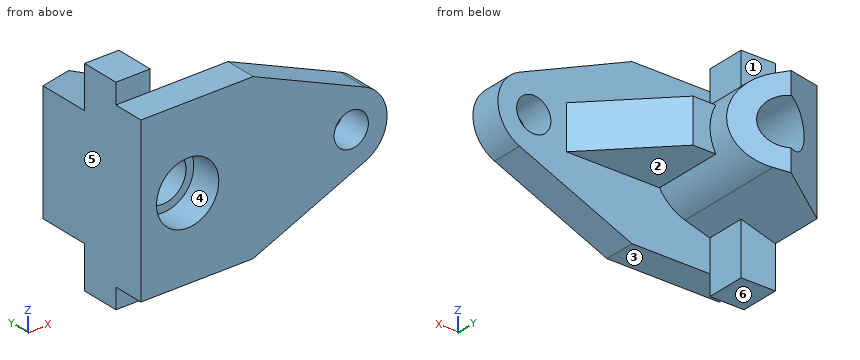
from build123d import *

# Parameters (mm, degrees)
BOSS_EXTRUDE2_DEPTH = 10
SKETCH2_R           = 5.5
CUT_EXTRUDE1_DEPTH  = 10
SKETCH3_W           = 11
SKETCH3_H           = 65
BOSS_EXTRUDE3_DEPTH = 12.5
BOSS_EXTRUDE4_START = -10
BOSS_EXTRUDE4_DEPTH = 47.5
SKETCH7_R           = 7.5
CUT_EXTRUDE2_DEPTH  = 89.705974996
RIB1_START          = -7
RIB1_DEPTH          = 14
CUT_EXTRUDE3_START  = -19
CUT_EXTRUDE3_DEPTH  = 38


# Read off the part's stored shape, not the designer's step: Rib1, Cut-Extrude3
with BuildPart() as part:
    # Sketch1 → Boss-Extrude2 (new body)
    with BuildSketch(Plane(origin=(0, 0, 0), x_dir=(1, 0, 0), z_dir=(0, 1, 0))):
        with BuildLine():
            Line((-67.5, 26), (-67.5, -26))
            Line((-67.5, -26), (-31.5, -26))
            Line((-31.5, -26), (4.527189528, -10.571402697))
            ThreePointArc((4.527189528, -10.571402697), (11.5, 0), (4.527189528, 10.571402697))
            Line((4.527189528, 10.571402697), (-31.5, 26))
            Line((-31.5, 26), (-67.5, 26))
        make_face()
    extrude(amount=BOSS_EXTRUDE2_DEPTH)

    # Sketch2 → Cut-Extrude1 (cut)
    with BuildSketch(Plane(origin=(0, 10, 0), x_dir=(1, 0, 0), z_dir=(0, 1, 0))):
        with Locations(Location((0, 0, 0), (0, 0, 270))):
            Circle(SKETCH2_R)
    extrude(amount=-CUT_EXTRUDE1_DEPTH, mode=Mode.SUBTRACT)

    # Sketch3 → Boss-Extrude3 (add)
    with BuildSketch(Plane(origin=(0, 10, 0), x_dir=(1, 0, 0), z_dir=(0, 1, 0))):
        with Locations((-62, 0)):
            Rectangle(SKETCH3_W, SKETCH3_H)
    extrude(amount=BOSS_EXTRUDE3_DEPTH)

    # Sketch4 → Boss-Extrude4 (add)
    with BuildSketch(Plane(origin=(0, 10, 0), x_dir=(1, 0, 0), z_dir=(0, 1, 0)).offset(BOSS_EXTRUDE4_START)):
        with BuildLine():
            Line((-67.5, 19), (-67.5, -19))
            Line((-67.5, -19), (-48.552766046, -13.432026806))
            ThreePointArc((-48.552766046, -13.432026806), (-38.5, 0), (-48.552766046, 13.432026806))
            Line((-48.552766046, 13.432026806), (-67.5, 19))
        make_face()
    extrude(amount=BOSS_EXTRUDE4_DEPTH)

    # Sketch6 → Hole1 (revolve, cut)
    with BuildSketch(Plane(origin=(-52.5, 10, 0), x_dir=(0, 0, 1), z_dir=(1, 0, 0))):
        Polygon((0, 0), (0, 10), (7, 10), (7, 15), (10, 15), (10, 0), align=None)
    revolve(axis=Axis((-52.5, -100, 0), (0, 1, 0)), mode=Mode.SUBTRACT)

    # Sketch7 → Cut-Extrude2 (cut, through all)
    with BuildSketch(Plane(origin=(0, 47.5, 0), x_dir=(1, 0, 0), z_dir=(0, 1, 0))):
        with Locations(Location((-52.5, 0, 0), (0, 0, 270))):
            Circle(SKETCH7_R)
    extrude(amount=-CUT_EXTRUDE2_DEPTH, mode=Mode.SUBTRACT)

    # Rib1 outline → Rib1 (add)
    with BuildSketch(Plane.XY.offset(RIB1_START)):
        Polygon((-33, 32.5), (-42, 32.5), (-42, 10), (-10.5, 10), align=None)
    extrude(amount=RIB1_DEPTH)

    # Cut-Extrude3 outline → Cut-Extrude3 (cut)
    with BuildSketch(Plane.XY.offset(CUT_EXTRUDE3_START)):
        Polygon((-37, 47.5), (-52.5, 47.5), (-38.5, 39.135888498), (-37, 38.239733694), align=None)
        Polygon((-67.5, 39.135888498), (-52.5, 47.5), (-67.5, 47.5), align=None)
    extrude(amount=CUT_EXTRUDE3_DEPTH, mode=Mode.SUBTRACT)


solid = part.part
CAD build for the part. Positions are in the model's coordinates, mm. Face numbers are marked on the shaded views. A direction names the side the tool comes from. Coordinates: 2 decimals unless noted, no trailing zeros. Order: outer loops, then holes, each group sorted by start corner. A loop starts at its lowest first (then second) coordinate and runs counter-clockwise, first axis right, second up.
Item 1: 3-axis set-ups, long thin cutter, end or side, ignore diameter. For the marked faces 1, 2 and 3: which of +Z, -Z, +X, -X, +Y, -Y reach the whole face in a straight line?
Check sheet entries:
face 1: +Z, +X, +Y
face 2: -Z, +X, +Y
face 3: -Z, +X, -X, -Y
Item 2: Band-saw the part on A-A on y = 31. List the corners of the cut face in (x, z), plus the area to 3 significant figures.
Check sheet entries:
outline: (-67.5, -19) - (-48.55, -13.43) arc R14 ccw to (-40.38, -7) - (-31.5, -7) - (-31.5, 7) - (-40.38, 7) arc R14 ccw to (-48.55, 13.43) - (-67.5, 19) - close; hole circle Ø15 at (-52.5, 0)
area: 743 mm2
Item 3: Drill centre lines: L1, parallel to X at y = 6.25, z = 0; L2, parallel to Z at x = -52.5, y = 36.5; L3, parallel to X at y = 37, z = 0. Where is each one in solid material? Low to high.
Check sheet entries:
L1: x = -67.5 to -62.5, -42.5 to -5.5, 5.5 to 11.5
L2: z = -14.59 to -7.5, 7.5 to 14.59
L3: x = -67.5 to -60, -45 to -38.5
Item 4: Pin check, flat tips, straight feed: pin 1 Ø10 at (y, z) = (16, -23.5) entering from +X; pin 2 Ø11 at (x, y) = (-24.5, 18.5) entering from -Z; pin 3 Ø8 at (x, z) = (-2.5, -17.5) entering from -Y; pin 4 Ø1 at (x, y) = (-37, 6.5) entering from +Z. Stop position of each tip, or through.
Check sheet entries:
pin 1: stops at x = -56.5
pin 2: stops at z = -7
pin 3: stops at y = 0
pin 4: stops at z = 26
Item 5: Band-saw the part on B-B on x = -2.5. List the corners of the cut face in (y, z), plus the area to 3 significant figures.
Check sheet entries:
outline: (0, -13.58) - (10, -13.58) - (10, -4.9) - (0, -4.9) - close; (0, 4.9) - (10, 4.9) - (10, 13.58) - (0, 13.58) - close
area: 174 mm2
Item 6: Band-saw the part on C-C on y = 4. List the corners of the cut face in (x, z), plus the area to 3 significant figures.
Check sheet entries:
outline: (-67.5, -26) - (-31.5, -26) - (4.53, -10.57) arc R11.5 ccw to (4.53, 10.57) - (-31.5, 26) - (-67.5, 26) - close; hole circle Ø20 at (-52.5, 0); hole circle Ø11 at (0, 0)
area: 2,890 mm2
Item 7: Two-plate mould, pull along Z, no slides. Class the marked faces 4, 5 and 6: +Z half, -Z half, draft (parallel to the pull), parting line (faces both ways), or undercut.
Check sheet entries:
face 4: undercut
face 5: draft
face 6: -Z half
Item 8: Band-saw the part on D-D on z = -20. List the corners of the cut face in (x, y), plus the area to 3 significant figures.
Check sheet entries:
outline: (-67.5, 0) - (-17.49, 0) - (-17.49, 10) - (-56.5, 10) - (-56.5, 22.5) - (-67.5, 22.5) - close
area: 638 mm2
